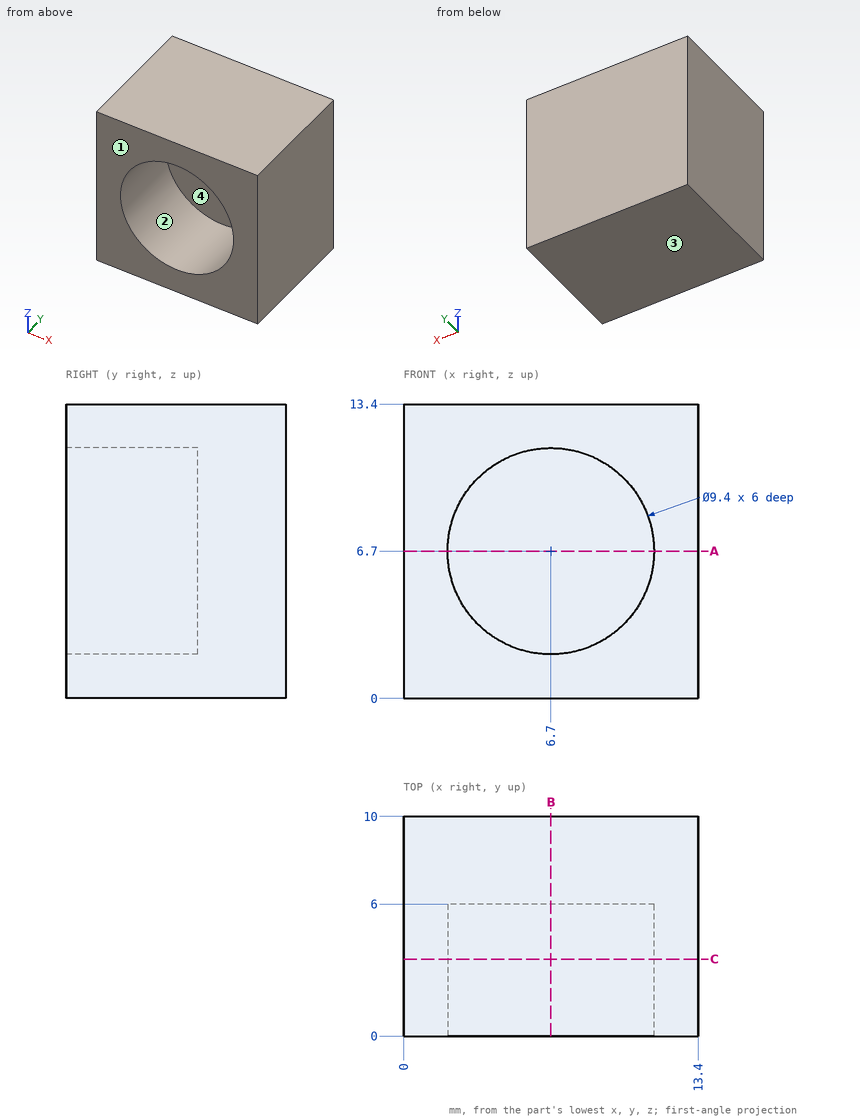
Drawing for the job (mm, zero at the part's lowest x, y, z). Round coordinates to 2 decimals unless told otherwise and drop trailing zeros. Order: outer loops, then holes, each group sorted by start corner. A loop starts at its lowest first (then second) coordinate and runs counter-clockwise, first axis right, second up. Notation, with made-up numbers: (39.5, 19.5) -> (95.5, 19.5) arc R27 ccw to (95.5, 47.5) -> close; hole circle Ø7 at (62.5, 86.25). An arc over 180 degrees is marked (long way). Write item = value, one per line. Start each with the question number.
(1) Probe line 1 (X direction, y = 2.75, z = 6.7); line 2 (Z direction, x = 3.5, y = 3). List the from-to ranges inside material, lowest first. Write a range as [from, to].
(2) Cut at C-C, the plane y = 3.5. List the corners of the cut face in (x, z), then the cut area to 3 significant figures.
(3) Cut at B-B, the plane x = 6.7. List the corners of the cut face in (y, z).
(4) Pull direction Z, two halves, no side cores. Call the marked faces 1, 2, 3 and 4: released by +Z, released by -Z, zero draft, split by the parting line, or undercut.
(5) Pin check, flat tip, straight feed: P1, Ø4, axis at x = 6, z = 5, coming from the -Y side. Stop position of the tip, or through.
(6) Cut at A-A, the plane z = 6.7. List the corners of the cut face in (x, y), then the cut area to 3 significant figures.
Model answer:
q1.line_1 = [0, 2], [11.4, 13.4]
q1.line_2 = [0, 3.26], [10.14, 13.4]
q2.outline = (0, 0) -> (13.4, 0) -> (13.4, 13.4) -> (0, 13.4) -> close; hole circle Ø9.4 at (6.7, 6.7)
q2.area = 110 mm2
q3.outline = (0, 0) -> (10, 0) -> (10, 13.4) -> (0, 13.4) -> (0, 11.4) -> (6, 11.4) -> (6, 2) -> (0, 2) -> close
q4.face_1 = zero draft
q4.face_2 = undercut
q4.face_3 = released by -Z
q4.face_4 = undercut
q5.P1 = 6
q6.outline = (0, 0) -> (2, 0) -> (2, 6) -> (11.4, 6) -> (11.4, 0) -> (13.4, 0) -> (13.4, 10) -> (0, 10) -> close
q6.area = 77.6 mm2
